Work out the finished part from the listing and answer in its coordinate system (mm). Face numbers are marked on the shaded views. A direction names the side the tool comes from. Round coordinates to 2 decimals unless told otherwise and drop trailing zeros. Loops run counter-clockwise (first coordinate to the right, second up) from the corner with the lowest first, then second, coordinate; pieces in that order, holes last.
```python
from build123d import *

# Parameters (mm, degrees)
F0_W      = 63.5
F0_H      = 12.7
F1_DEPTH  = 50.8
F2_W      = 50.7968105376
F2_H      = 12.6984052688
F3_DEPTH  = 50.8
F5_DEPTH  = 50.8
F6_W      = 25.3984052688
F6_H      = 25.4
F7_DEPTH  = 12.7
F8_W      = 12.6992026344
F8_H      = 25.4
F9_DEPTH  = 12.7
F10_W     = 13.0463411808
F10_H     = 26.8100267276
F11_DEPTH = 12.7
F13_DEPTH = 12.7
F15_DEPTH = 12.7
F16_R     = 6.3492026344
F17_DEPTH = 38.1


with BuildPart() as f1:
    # F0 (on Front) → F1 (new body)
    with BuildSketch(Plane.XZ):
        with Locations((31.75, 6.35)):
            Rectangle(F0_W, F0_H)
    extrude(amount=F1_DEPTH)

    # F2 (on face) → F3 (join)
    with BuildSketch(Plane.XZ.offset(50.8)):
        with Locations((25.3984052688, 19.0492026344)):
            Rectangle(F2_W, F2_H)
    extrude(amount=-F3_DEPTH)

    # F4 (on face) → F5 (join)
    with BuildSketch(Plane.XZ.offset(50.8)):
        Polygon((0, 38.0984052688), (0, 25.3984052688), (25.3984052688, 25.3984052688), (25.3984052688, 50.7984052688), (12.6490090042, 50.7984052688), align=None)
    extrude(amount=-F5_DEPTH)

    # F6 (on face) → F7 (join)
    with BuildSketch(Plane.XY.offset(25.3984052688)):
        with Locations((38.0976079032, -25.6369028568)):
            Rectangle(F6_W, F6_H)
    extrude(amount=F7_DEPTH)

    # F8 (on face) → F9 (join)
    with BuildSketch(Plane.XY.offset(38.0984052688)):
        with Locations((31.748006586, -25.6369028568)):
            Rectangle(F8_W, F8_H)
    extrude(amount=F9_DEPTH)

    # F10 (on face) → F11 (join)
    with BuildSketch(Plane.XY.offset(12.7)):
        with Locations((70.0231705904, -24.706099648)):
            Rectangle(F10_W, F10_H)
    extrude(amount=-F11_DEPTH)

    # F12 (on face) → F13 (join)
    with BuildSketch(Plane.XY.offset(12.7)):
        with BuildLine():
            Line((63.5, -11.3010862842), (76.5463411808, -11.3010862842))
            ThreePointArc((76.5463411808, -11.3010862842), (72.1302023355, -3.2181172377), (63.5, 0))
            Line((63.5, 0), (63.5, -11.3010862842))
        make_face()
    extrude(amount=-F13_DEPTH)

    # F14 (on face) → F15 (join)
    with BuildSketch(Plane.XY.offset(12.7)):
        with BuildLine():
            Line((63.5, -38.1111130118), (63.5, -50.8))
            ThreePointArc((63.5, -50.8), (72.7010118925, -47.2088343378), (76.5463411808, -38.1111130118))
            Line((76.5463411808, -38.1111130118), (63.5, -38.1111130118))
        make_face()
    extrude(amount=-F15_DEPTH)

    # F16 (on face) → F17 (cut, symmetric)
    with BuildSketch(Plane.YZ.offset(50.7968105376)):
        with Locations((-25.4, 12.7)):
            Circle(F16_R)
    extrude(amount=F17_DEPTH, both=True, mode=Mode.SUBTRACT)


solid = f1.part
```
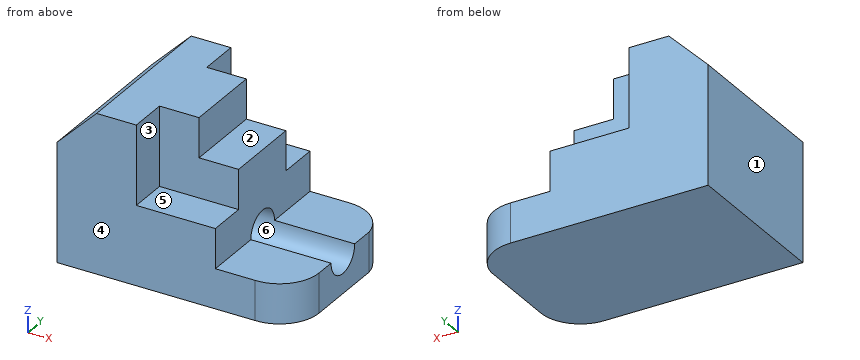
1. Find section A-A (y = -25.4). Write down the section's boundary in (x, z).
Answer key:
outline: (0, 0) - (76.55, 0) - (76.55, 6.35) - (12.7, 6.35) - (12.7, 19.05) - (50.8, 19.05) - (50.8, 38.1) - (38.1, 38.1) - (38.1, 50.8) - (12.65, 50.8) - (0, 38.1) - close
2. Find section D-D (z = 21.5). Write down the section's boundary in (x, y), then the cut area to 3 significant figures.
Answer key:
outline: (0, -50.8) - (50.8, -50.8) - (50.8, 0) - (0, 0) - close
area: 2,580 mm2
3. Given pin 1 (6 mm diameter, centred on y = -44, z = 32.5, fed in from +X); pin 2 (7.5 mm diameter, centred on y = -25.4, z = 12.7, fed in from +X); pin 3 (3.5 mm diameter, centred on x = 38, y = -43.5, fed in from +Z), each flat-ended and moving along its own axis, determine where each tip first touches the part or whether it passes through.
Answer key:
pin 1: stops at x = 25.4
pin 2: stops at x = 12.7
pin 3: stops at z = 25.4
4. Determine the mould class of the marked faces 4, 5 and 6 for opening direction Z: +Z half, -Z half, draft (parallel to the pull), parting line (faces both ways), or undercut.
Answer key:
face 4: draft
face 5: +Z half
face 6: undercut
5. Find section B-B (z = 10). Write down the section's boundary in (x, y), then the cut area to 3 significant figures.
Answer key:
outline: (0, -50.8) - (63.5, -50.8) arc R12.7 ccw to (76.55, -38.11) - (76.55, -31.15) - (12.7, -31.15) - (12.7, -19.65) - (76.55, -19.65) - (76.55, -11.3) arc R13.18 ccw to (63.5, 0) - (0, 0) - close
area: 3,080 mm2
6. Find section C-C (y = -35). Write down the section's boundary in (x, z), then the cut area to 3 significant figures.
Answer key:
outline: (0, 0) - (76.55, 0) - (76.55, 12.7) - (50.8, 12.7) - (50.8, 38.1) - (38.1, 38.1) - (38.1, 50.8) - (12.65, 50.8) - (0, 38.1) - close
area: 2,670 mm2
7. Which of the six approach directions +Z, -Z, +X, -X, +Y, -Y give full straight-line access (tool end or side, diameter ignored) to the marked faces 1, 2 and 3?
Answer key:
face 1: +Z, -Z, -X, +Y, -Y
face 2: +Z, +X, +Y, -Y
face 3: +Z, +X, -Y
8. Consider probe 1 along Z at (x, y) = (49, -25); probe 2 along Z at (x, y) = (31.5, -25.4); probe 3 along X at (y, z) = (-32, 32). Determine where each line is inside the solid, lowest interval first.
Answer key:
probe 1: z = 0 to 6.36, 19.04 to 38.1
probe 2: z = 0 to 6.35, 19.05 to 50.8
probe 3: x = 0 to 50.8
